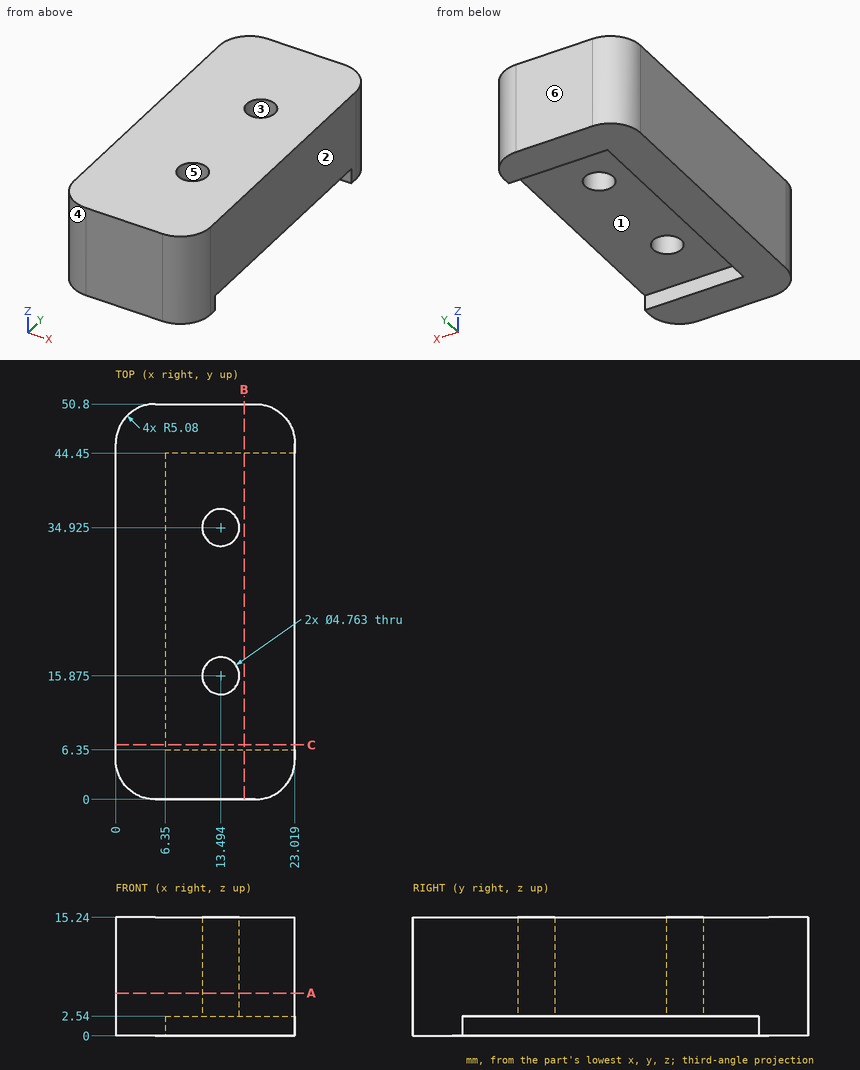
For this review, use the dimensioned drawing (mm, ordinates from the lowest corner) and the shaded views. A direction names the side the tool comes from. Give positions to 0.01 mm unless a question says otherwise; leave off trailing zeros. Order: outer loops, then holes, each group sorted by start corner. A loop starts at its lowest first (then second) coordinate and runs counter-clockwise, first axis right, second up.
1) The part is to be moulded in two halves that separate along X. For the marked faces 3, 4, 5 and 6, say which applies: released by +X, released by -X, zero draft, split by the parting line, or undercut.
2) Take a section at C-C (y = 7). Give the boundary of the cut face in (x, z).
3) Wall thickness on line 1 (Y direction, x = 14.75, z = 8); line 2 (Y direction, x = 15.5, z = 7.5) (1 decimal); line 3 (Z direction, x = 10.5, y = 25): over which ranges is each line inside the solid? List them lowest first.
4) Insertion check: pin 1 (3 mm diameter, centred on x = 8.5, y = 37, fed in from -Z); pin 2 (3 mm diameter, centred on y = 22, z = 1, fed in from +X); pin 3 (5.5 mm diameter, centred on x = 13.49, y = 34.93, fed in from +Z). Each pin has a flat end and moves straight along its axis. Give the tip position at first contact, or say it passes through.
5) Take a section at B-B (x = 16.5). Give the boundary of the cut face in (y, z).
6) For the marked faces 1 and 2, list the 3-axis set-ups (+Z, -Z, +X, -X, +Y, -Y) from which the entire face can be reached by the end or side of a thin tool; tool diameter is ignored.
7) Take a section at A-A (z = 5.5). Give the boundary of the cut face in (x, y) (1 decimal).
Derived:
1. face 3: undercut
1. face 4: released by -X
1. face 5: undercut
1. face 6: zero draft
2. outline: (0, 0) - (6.35, 0) - (6.35, 2.54) - (23.02, 2.54) - (23.02, 15.24) - (0, 15.24) - close
3. line 1: y = 0 to 13.85, 17.9 to 32.9, 36.95 to 50.8
3. line 2: y = 0 to 14.6, 17.2 to 33.6, 36.2 to 50.8
3. line 3: z = 2.54 to 15.24
4. pin 1: stops at z = 2.54
4. pin 2: stops at x = 6.35
4. pin 3: stops at z = 15.24
5. outline: (0, 0) - (6.35, 0) - (6.35, 2.54) - (44.45, 2.54) - (44.45, 0) - (50.8, 0) - (50.8, 15.24) - (0, 15.24) - close
6. face 1: -Z, +X
6. face 2: +Z, -Z, +X, +Y, -Y
7. outline: (0, 5.1) arc R5.1 ccw to (5.1, 0) - (17.9, 0) arc R5.1 ccw to (23, 5.1) - (23, 45.7) arc R5.1 ccw to (17.9, 50.8) - (5.1, 50.8) arc R5.1 ccw to (0, 45.7) - close; hole circle Ø4.8 at (13.5, 15.9); hole circle Ø4.8 at (13.5, 34.9)
